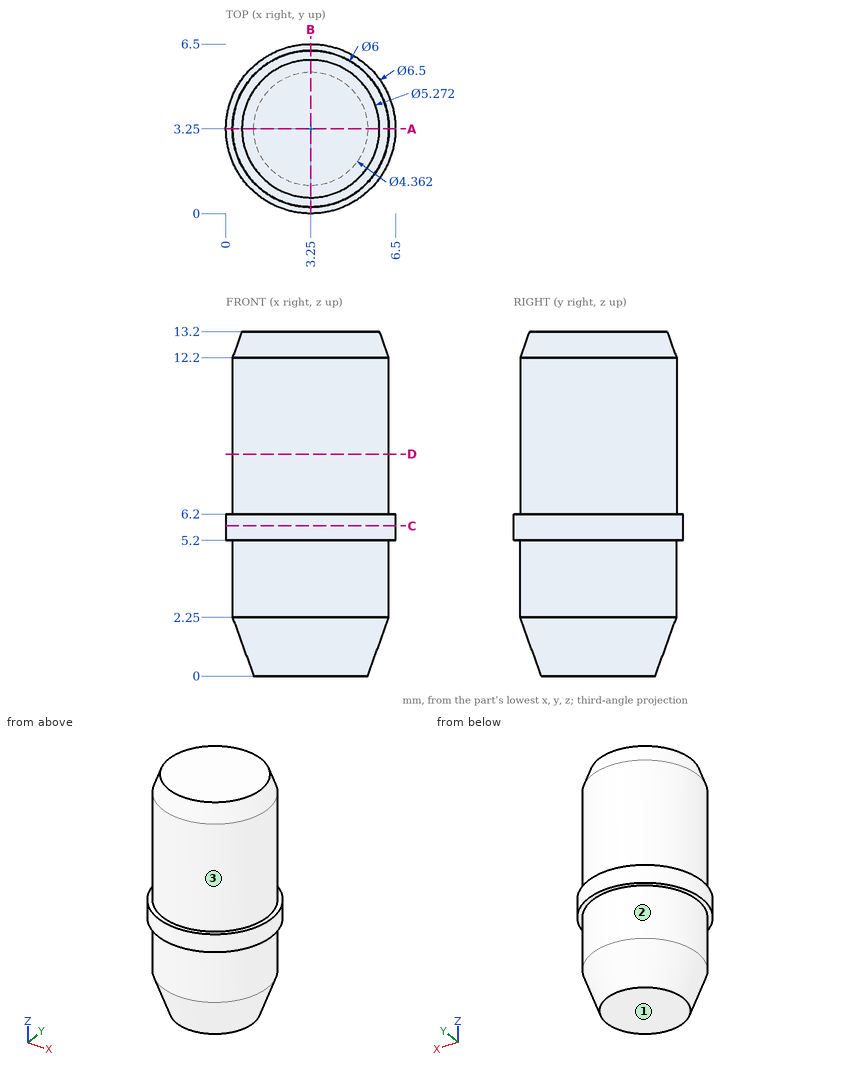
Input: dimensioned drawing with shaded views. Units: mm. Origin: part minimum x, y, z. A direction names the side the tool comes from. Round coordinates to 2 decimals unless told otherwise and drop trailing zeros. Loops run counter-clockwise (first coordinate to the right, second up) from the corner with the lowest first, then second, coordinate; pieces in that order, holes last. Notation, with made-up numbers: (50, 74) -> (82, 74) arc R25 ccw to (82, 92) -> close; hole circle Ø6 at (75, 26). An arc over 180 degrees is marked (long way). Use one line per item in the form item = value. Start each with the question number.
1) Section D-D on z = 8.5. Output: boundary loops of the cut face in (x, y), then the cut area to 3 significant figures.
2) Section C-C on z = 5.75. Output: boundary loops of the cut face in (x, y), then the cut area to 3 significant figures.
3) Line query: L1, parallel to Y at x = 3.25, z = 3; L2, parallel to Z at x = 0.75, y = 5.25; L3, parallel to Y at x = 4.5, z = 1.75. Output: solid intervals per line, ascending.
4) First-contact query: P1, Ø1.5, axis at y = 4, z = 10, coming from the +X side; P2, Ø1.5, axis at x = 3, z = 8, coming from the +Y side. Flat tips, straight axial feed; report the tip coordinate or a pass-through.
5) Access query for the marked faces 1, 2 and 3. Directions: +Z, -Z, +X, -X, +Y, -Y. A direction counts if a zero-diameter tool reaches every point of the face in a straight line with its end or side. Return the directions, or none.
6) Section A-A on y = 3.25. Output: boundary loops of the cut face in (x, z).
Response:
q1.outline = circle Ø6 at (3.25, 3.25)
q1.area = 28.3 mm^2
q2.outline = circle Ø6.5 at (3.25, 3.25)
q2.area = 33.2 mm^2
q3.L1 = 0.25 to 6.25
q3.L2 = 5.2 to 6.2
q3.L3 = 0.72 to 5.78
q4.P1 = 6.25
q4.P2 = 6.25
q5.face_1 = -Z, +X, -X, +Y, -Y
q5.face_2 = -Z
q5.face_3 = +Z
q6.outline = (0, 5.2) -> (0.25, 5.2) -> (0.25, 2.25) -> (1.07, 0) -> (5.43, 0) -> (6.25, 2.25) -> (6.25, 5.2) -> (6.5, 5.2) -> (6.5, 6.2) -> (6.25, 6.2) -> (6.25, 12.2) -> (5.89, 13.2) -> (0.61, 13.2) -> (0.25, 12.2) -> (0.25, 6.2) -> (0, 6.2) -> close
